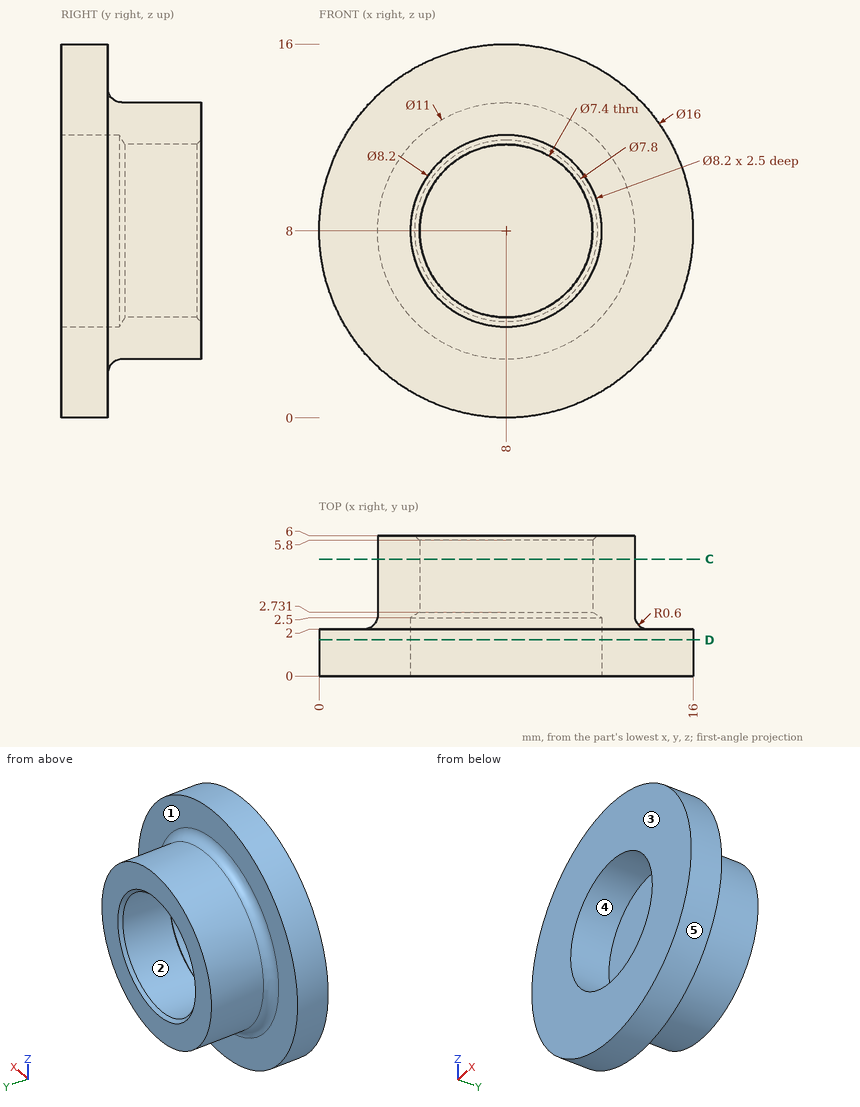
Print and shaded views of the part. All mm, measured from the part's lowest x, y and z. A direction names the side the tool comes from. Give positions to 0.01 mm unless a question says otherwise; leave off trailing zeros. Loops run counter-clockwise (first coordinate to the right, second up) from the corner with the lowest first, then second, coordinate; pieces in that order, holes last. Notation, with made-up numbers: (-16, -3) - (-4, -3) arc R21 cw to (-4, 17) - close; hole circle Ø1 at (42.25, -19). An arc over 180 degrees is marked (long way). Use a Markdown table: item, result.
(1) Drop flat-ended pins along their axis: pin 1 Ø2.5 at (x, z) = (6.5, 9.5) entering from -Y; pin 2 Ø3 at (x, y) = (11, 5) entering from +Z; pin 3 Ø2 at (x, y) = (6.5, 5) entering from +Z. Give the stop position or say it passes through.
Taken from the geometry:
| item | result |
|---|---|
| pin 1 | through |
| pin 2 | z = 13.29 |
| pin 3 | z = 13.48 |
(2) Band-saw the part on C-C (y = 5). Give the cut face in (x, z).
Taken from the geometry:
| item | result |
|---|---|
| outline | circle Ø11 at (8, 8); hole circle Ø7.4 at (8, 8) |
(3) Pull direction X, two halves, no side cores. Call the marked faces 3, 4 and 5: +X half, -X half, draft (parallel to the pull), parting line (faces both ways), or undercut.
Taken from the geometry:
| item | result |
|---|---|
| face 3 | draft |
| face 4 | undercut |
| face 5 | parting line |
(4) Band-saw the part on D-D (y = 1.55). Give the cut face in (x, z).
Taken from the geometry:
| item | result |
|---|---|
| outline | circle Ø16 at (8, 8); hole circle Ø8.2 at (8, 8) |
(5) Which spindle directions (+Z, -Z, +X, -X, +Y, -Y) get a long thin tool onto all of the face, cutting with end or side? Do the marked faces 1 and 2. Say none if no direction does.
Taken from the geometry:
| item | result |
|---|---|
| face 1 | +Y |
| face 2 | +Y, -Y |
(6) Wall check: line 1 along X through (y, z) = (3.85, 8); line 2 along X through (y, z) = (1.35, 8); line 3 along Y through (x, z) = (13.5, 5.5). Give the ranges that are in metal, low to high.
Taken from the geometry:
| item | result |
|---|---|
| line 1 | 2.5 to 4.3, 11.7 to 13.5 |
| line 2 | 0 to 3.9, 12.1 to 16 |
| line 3 | 0 to 2 |
